from build123d import *

# Parameters (mm, degrees)
SKETCH1_R                = 40
BOSS_EXTRUDE1_DEPTH      = 2
SKETCH4_R                = 3
BOSS_EXTRUDE3_DEPTH      = 2
FILLET2_R                = 4
CIRPATTERN2_COUNT        = 3
FILLET2_OF_CIRPATTERN2_R = 4
SKETCH5_R                = 10
CUT_EXTRUDE1_DEPTH       = 8
CUT_EXTRUDE3_DEPTH       = 15
FILLET3_R                = 5
CIRPATTERN4_COUNT        = 3
FILLET3_OF_CIRPATTERN4_R = 5
SKETCH6_R                = 2
CUT_EXTRUDE4_DEPTH       = 10
CIRPATTERN5_COUNT        = 4


with BuildPart() as part:
    # Sketch1 → Boss-Extrude1 (new body)
    with BuildSketch(Plane.XY):
        Circle(SKETCH1_R)
    extrude(amount=BOSS_EXTRUDE1_DEPTH)

    # Sketch4 → Boss-Extrude3 (add)
    with BuildSketch(Plane(origin=(0, 0, 0), x_dir=(-1, 0, 0), z_dir=(0, 0, -1))):
        with BuildLine():
            Line((-15.513007814, 36.869317712), (-18.669872981, 42.337168574))
            ThreePointArc((-18.669872981, 42.337168574), (-25.5, 44.167295593), (-27.330127019, 37.337168574))
            Line((-27.330127019, 37.337168574), (-24.173261852, 31.869317712))
            Line((-24.173261852, 31.869317712), (-15.513007814, 36.869317712))
        make_face()
        with Locations((-23, 39.837168574)):
            Circle(SKETCH4_R, mode=Mode.SUBTRACT)
    boss_extrude3 = extrude(amount=-BOSS_EXTRUDE3_DEPTH)

    # Fillet2
    fillet2_edges = [part.edges().sort_by_distance(p)[0] for p in [
        (15.513007814, 36.869317712, 1),
        (24.173261852, 31.869317712, 1),
    ]]
    fillet(fillet2_edges, radius=FILLET2_R)

    # CirPattern2: Boss-Extrude3 ×3 about axis
    cirpattern2_axis = Axis((0, 0, 0), (0, 0, 1))
    for i in range(1, CIRPATTERN2_COUNT):
        add(boss_extrude3.rotate(cirpattern2_axis, i * 360 / CIRPATTERN2_COUNT))

    # Fillet2 of CirPattern2
    fillet2_of_cirpattern2_edges = [part.edges().sort_by_distance(p)[0] for p in [
        (-39.686269666, -5, 1),
        (-39.686269666, 5, 1),
        (24.173261852, -31.869317712, 1),
        (15.513007814, -36.869317712, 1),
    ]]
    fillet(fillet2_of_cirpattern2_edges, radius=FILLET2_OF_CIRPATTERN2_R)

    # Sketch5 → Cut-Extrude1 (cut)
    with BuildSketch(Plane(origin=(0, 0, 0), x_dir=(-1, 0, 0), z_dir=(0, 0, -1))):
        Circle(SKETCH5_R)
    extrude(amount=-CUT_EXTRUDE1_DEPTH, mode=Mode.SUBTRACT)

    # Sketch7 → Cut-Extrude3 (cut)
    with BuildSketch(Plane(origin=(0, 0, 0), x_dir=(-1, 0, 0), z_dir=(0, 0, -1))):
        with BuildLine():
            ThreePointArc((-5.156603958, 19.323804895), (10, 17.320508076), (19.313207916, 5.196152423))
            Line((19.313207916, 5.196152423), (32.081926376, 5.196152423))
            ThreePointArc((32.081926376, 5.196152423), (16.25, 28.145825623), (-11.540963188, 30.381839455))
            Line((-11.540963188, 30.381839455), (-5.156603958, 19.323804895))
        make_face()
    cut_extrude3 = extrude(amount=-CUT_EXTRUDE3_DEPTH, mode=Mode.SUBTRACT)

    # Fillet3
    fillet3_edges = [part.edges().sort_by_distance(p)[0] for p in [
        (-32.081926376, 5.196152423, 1),
        (-19.313207916, 5.196152423, 1),
        (5.156603958, 19.323804895, 1),
        (11.540963188, 30.381839455, 1),
    ]]
    fillet(fillet3_edges, radius=FILLET3_R)

    # CirPattern4: Cut-Extrude3 ×3 about axis
    cirpattern4_axis = Axis((0, 0, 0), (0, 0, 1))
    for i in range(1, CIRPATTERN4_COUNT):
        add(cut_extrude3.rotate(cirpattern4_axis, i * 360 / CIRPATTERN4_COUNT), mode=Mode.SUBTRACT)

    # Fillet3 of CirPattern4
    fillet3_of_cirpattern4_edges = [part.edges().sort_by_distance(p)[0] for p in [
        (11.540963188, -30.381839455, 1),
        (5.156603958, -19.323804895, 1),
        (-19.313207916, -5.196152423, 1),
        (-32.081926376, -5.196152423, 1),
        (20.540963188, 25.185687033, 1),
        (14.156603958, 14.127652472, 1),
        (14.156603958, -14.127652472, 1),
        (20.540963188, -25.185687033, 1),
    ]]
    fillet(fillet3_of_cirpattern4_edges, radius=FILLET3_OF_CIRPATTERN4_R)

    # Sketch6 → Cut-Extrude4 (cut)
    with BuildSketch(Plane(origin=(0, 0, 0), x_dir=(-1, 0, 0), z_dir=(0, 0, -1))):
        with Locations((4.07639996, -15.213331764)):
            Circle(SKETCH6_R)
    cut_extrude4 = extrude(amount=-CUT_EXTRUDE4_DEPTH, mode=Mode.SUBTRACT)

    # CirPattern5: Cut-Extrude4 ×4 about axis
    cirpattern5_axis = Axis((0, 0, 0), (0, 0, 1))
    for i in range(1, CIRPATTERN5_COUNT):
        add(cut_extrude4.rotate(cirpattern5_axis, i * 360 / CIRPATTERN5_COUNT), mode=Mode.SUBTRACT)


solid = part.part
Read the model definition and answer for the solid it produces. Units are mm, in the model's axes. A direction names the side the tool comes from. Round coordinates to 2 decimals unless told otherwise and drop trailing zeros. Write each loop counter-clockwise with the first axis right and the second up, starting at its lowest first coordinate (ties: lowest second). Pieces come first, ordered by that corner, then holes.
1. Straight lines are drawn through the part: L1, parallel to X at y = -8, z = 1.75; L2, parallel to X at y = 9, z = 1.7; L3, parallel to Y at x = 23, z = 0.75. For each, find the intervals that lie inside material, in ascending order.
2. Determine the mould class of faces 4 (the face through (-11, 0, 0)), 5 (the face through (25.595, -44.111, 0.986)), 6 (the face through (17.95, -41.09, 0.99)) for opening direction Y: pulls with the +Y half, pulls with the -Y half, needs draft (parallel to the pull), parting line crosses it, or undercut.
3. Which of the six approach directions +Z, -Z, +X, -X, +Y, -Y give full straight-line access (tool end or side, diameter ignored) to faces 1 (the face through (-29.641, 7.335, 1.014)), 2 (the face through (26.587, -36.051, 0.986)), 3 (the face through (-40.52, 5.92, 1.01))?
4. The part is cut by section A-A, the plane x = 0. Determine the outline of the cut face in (y, z), then the cut area to 3 significant figures.
5. The part is cut by section B-B, the plane y = 0. Determine the outline of the cut face in (x, z).
6. Given pin 1 Ø1 at (x, z) = (-24, 0.5) entering from +Y; pin 2 Ø18 at (x, y) = (0, 0) entering from -Z; pin 3 Ø0.6 at (x, z) = (-44.5, 1) entering from +Y, each flat-ended and moving along its own axis, determine where each tip first touches the part or whether it passes through.
7. The part is cut by section C-C, the plane x = -28.5. Determine the outline of the cut face in (y, z), then the cut area to 3 significant figures.
8. The part is cut by section D-D, the plane z = 1.25. State how many separate pieces and enclosed holes the cut face has, then the cut area to 3 significant figures.
Values:
1. L1: x = -39.2 to -30.03, -18.33 to -6, 6 to 18.33, 31.5 to 39.19
1. L2: x = -38.97 to -30.39, -17.86 to -4.36, 4.36 to 17.86, 31.23 to 38.97
1. L3: y = -44.84 to -42.84, -36.84 to -21.82, 21.82 to 36.84, 42.84 to 44.84
2. face 4: needs draft
2. face 5: undercut
2. face 6: pulls with the -Y half
3. face 1: +Z, -Z
3. face 2: +Z, -Z, +X
3. face 3: +Z, -Z, -X, +Y
4. outline: (-40, 0) - (-32.5, 0) - (-32.5, 2) - (-40, 2) - close; (-20, 0) - (-10, 0) - (-10, 2) - (-20, 2) - close; (10, 0) - (20, 0) - (20, 2) - (10, 2) - close; (32.5, 0) - (40, 0) - (40, 2) - (32.5, 2) - close
4. area: 70.0 mm2
5. outline: (-51, 0) - (-49, 0) - (-49, 2) - (-51, 2) - close; (-43, 0) - (-10, 0) - (-10, 2) - (-43, 2) - close; (10, 0) - (20, 0) - (20, 2) - (10, 2) - close; (32.5, 0) - (40, 0) - (40, 2) - (32.5, 2) - close
6. pin 1: stops at y = 32.37
6. pin 2: passes through
6. pin 3: stops at y = 5
7. outline: (-28.07, 0) - (-15.62, 0) - (-15.62, 2) - (-28.07, 2) - close; (-6.17, 0) - (6.17, 0) - (6.17, 2) - (-6.17, 2) - close; (15.62, 0) - (28.07, 0) - (28.07, 2) - (15.62, 2) - close
7. area: 74.5 mm2
8. separate pieces: 1
8. enclosed holes: 11
8. area: 3,300 mm2
